Build history of the part. All positions in model axes, mm. Face numbers are marked on the shaded views. A direction names the side the tool comes from. Give positions to 0.01 mm unless a question says otherwise; leave off trailing zeros. Loops run counter-clockwise (first coordinate to the right, second up) from the corner with the lowest first, then second, coordinate; pieces in that order, holes last. Notation, with made-up numbers: M 48.25,18 L 64.25,18 A7 ccw 64.25,23 Z; hole C 33,75.5 d1. An arc over 180 degrees is marked long. Answer as a JSON object with one key per item and string values. Group by question number.
1. Mould opens along X. For the marked faces 3, 4, 5 and 6 say: released by +X, released by -X, zero draft, split by the parting line, or undercut.
2. Slice it at B-B (x = -31.5). List the corners of the cut face in (y, z) (3 decimals).
3. Drill centre lines: line 1 along Y through (x, z) = (-44, -1.75); line 2 along X through (y, z) = (-13, -16.5); line 3 along X through (y, z) = (22.5, -6.5). Where is each one in solid material? Low to high. Write a range as [from, to].
4. Slice it at D-D (y = 24). List the corners of the cut face in (x, z) (1 decimal), then the cut area to 3 significant figures.
5. Slice it at C-C (z = -2.75). List the corners of the cut face in (x, y), then the cut area to 3 significant figures.
6. Slice it at A-A (y = 0). List the corners of the cut face in (x, z), then the cut area to 3 significant figures.
7. 3-axis set-ups, long thin cutter, end or side, ignore diameter. For the marked faces 1 and 2: which of +Z, -Z, +X, -X, +Y, -Y reach the whole face in a straight line?
8. Drop flat-ended pins along their axis: pin 1 Ø19 at (x, y) = (-26.5, 17) entering from -Z (3 decimals); pin 2 Ø5.5 at (x, z) = (-40, -2) entering from +Y; pin 3 Ø5 at (y, z) = (-5, -16.5) entering from -X; pin 4 Ø3.5 at (y, z) = (0, -10.922) entering from -X. Give the stop position or say it passes through.
from build123d import *

# Parameters (mm, degrees)
BOSS_EXTRUDE1_DEPTH       = 22.606
CUT_EXTRUDE1_DEPTH        = 56.118
F_8_CLEARANCE_HOLE1_D     = 4.3053
F_8_CLEARANCE_HOLE1_DEPTH = 3.81
CHAMFER1_SIZE             = 16.51


with BuildPart() as part:
    # Sketch1 w/mock PCB → Boss-Extrude1 (new body)
    with BuildSketch(Plane.XY):
        with BuildLine():
            Line((-19.05, 18.923), (-50.292, 18.923))
            Line((-50.292, 18.923), (-50.292, 27.559))
            Line((-50.292, 27.559), (3.81, 27.559))
            Line((3.81, 27.559), (3.81, -27.559))
            Line((3.81, -27.559), (-50.292, -27.559))
            Line((-50.292, -27.559), (-50.292, -18.923))
            Line((-50.292, -18.923), (-19.05, -18.923))
            ThreePointArc((-19.05, -18.923), (-0.127, 0), (-19.05, 18.923))
        make_face()
    extrude(amount=-BOSS_EXTRUDE1_DEPTH)

    # Sketch1 → Cut-Extrude1 (cut, through all)
    with BuildSketch(Plane.XZ.offset(27.559)):
        Polygon((-3.302, -5.08), (-3.302, -1.905), (-43.18, -1.905), (-43.18, -5.08), (-50.292, -5.08), (-50.292, -22.606), (0, -22.606), (0, -5.08), align=None)
    extrude(amount=-CUT_EXTRUDE1_DEPTH, mode=Mode.SUBTRACT)

    # #8 Clearance Hole1
    with Locations(Plane(origin=(3.81, 0, 0), x_dir=(0, 0, -1), z_dir=(1, 0, 0))):
        with Locations((10.922, 0)):
            Hole(F_8_CLEARANCE_HOLE1_D / 2, depth=F_8_CLEARANCE_HOLE1_DEPTH)

    # Sketch8 → Revolve1 (revolve)
    with BuildSketch(Plane(origin=(0, 23.241, 0), x_dir=(1, 0, 0), z_dir=(0, 1, 0))):
        with BuildLine():
            Line((-46.736, 8.0518), (-46.736, 5.08))
            Line((-46.736, 5.08), (-44.577, 5.08))
            Line((-44.577, 5.08), (-44.577, 7.673501516))
            ThreePointArc((-44.577, 7.673501516), (-45.640053977, 7.95651041), (-46.736, 8.0518))
        make_face()
    revolve1 = revolve(axis=Axis((-46.736, 23.241, -5.08), (0, 0, 1)))

    # Mirror1: Revolve1 across plane
    add(revolve1.mirror(Plane.ZX))

    # Chamfer1
    chamfer1_edges = [part.edges().sort_by_distance(p)[0] for p in [
        (1.905, -27.559, -22.606),
        (1.905, 27.559, -22.606),
    ]]
    chamfer(chamfer1_edges, length=CHAMFER1_SIZE)


solid = part.part
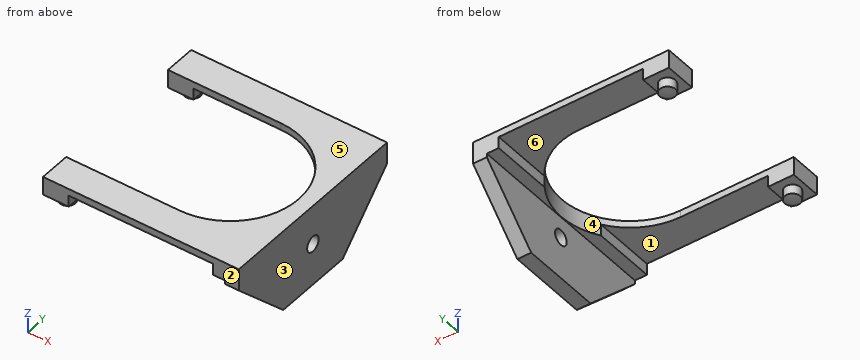
Established:
{
 "1": {"face 3": "released by +X", "face 4": "released by -X", "face 5": "zero draft", "face 6": "undercut"},
 "2": {"outline": "M -27.559,-1.905 L -18.923,-1.905 L -18.923,0 L -27.559,0 Z; M 18.923,-1.905 L 27.559,-1.905 L 27.559,0 L 18.923,0 Z"},
 "3": {"line 1": "y = [-27.56, -18.92], [18.92, 27.56]", "line 2": "x = [0, 3.81]", "line 3": "x = [-48.76, -44.71], [0, 3.81]"},
 "4": {"outline": "M -50.3,-5.1 L -48.8,-5.1 L -48.8,-7.7 A6.3 ccw -44.7,-7.7 L -44.7,-5.1 L -43.2,-5.1 L -43.2,-1.9 L -3.3,-1.9 L -3.3,-5.1 L 0,-5.1 L 0,-9.7 L 3.8,-9.7 L 3.8,0 L -50.3,0 Z", "area": "177 mm^2"},
 "5": {"outline": "M -50.29,-27.56 L -43.18,-27.56 L -43.18,-18.92 L -50.29,-18.92 Z; M -50.29,18.92 L -43.18,18.92 L -43.18,27.56 L -50.29,27.56 Z; M -3.3,-27.56 L 3.81,-27.56 L 3.81,27.56 L -3.3,27.56 L -3.3,10.49 A18.92 cw -3.3,-10.49 Z", "area": "470 mm^2"},
 "6": {"outline": "M -0.13,-5.08 L 0,-5.08 L 0,-8.77 L 3.81,-8.77 L 3.81,0 L -0.13,0 Z; M 0,-22.61 L 3.81,-22.61 L 3.81,-13.07 L 0,-13.07 Z", "area": "70.4 mm^2"},
 "7": {"face 1": "-Z, +Y, -Y", "face 2": "+Z, -Z, +X, -X, -Y"},
 "8": {"pin 1": "stops at z = -1.905", "pin 2": "stops at y = 27.56", "pin 3": "stops at x = 0", "pin 4": "passes through"}
}
